from build123d import *

# Parameters (mm, degrees)
F0_W     = 19.05
F0_H     = 10.024884
F0_R     = 3.2004
F1_DEPTH = 25.4
F2_DEPTH = 19.05
F3_DEPTH = 25.4


with BuildPart() as f1:
    # F0 (on Front) → F1 (new body)
    with BuildSketch(Plane.XZ):
        with Locations((47.891052, 14.037558)):
            Rectangle(F0_W, F0_H)
        Polygon((19.316052, 0), (171.716052, 0), (171.716052, 19.05), (57.416052, 19.05), (57.416052, 9.025116), (38.366052, 9.025116), (38.366052, 19.05), (19.316052, 19.05), align=None)
        with Locations((159.016052, 10.429697)):
            Circle(F0_R, mode=Mode.SUBTRACT)
    extrude(amount=F1_DEPTH)

    # F0 (on Front) → F2 (join)
    with BuildSketch(Plane.XZ):
        with Locations((47.891052, 14.037558)):
            Rectangle(F0_W, F0_H)
    extrude(amount=F2_DEPTH)

    # F0 (on Front) → F3 (cut)
    with BuildSketch(Plane.XZ):
        with Locations((47.891052, 14.037558)):
            Rectangle(F0_W, F0_H)
    extrude(amount=F3_DEPTH, mode=Mode.SUBTRACT)


solid = f1.part
Source: CAD feature listing. Evaluate the final solid. Frame: model axes, mm. A direction names the side the tool comes from. Round coordinates to 2 decimals unless told otherwise and drop trailing zeros. Write each loop counter-clockwise with the first axis right and the second up, starting at its lowest first coordinate (ties: lowest second). Pieces come first, ordered by that corner, then holes. Notation, with made-up numbers: (76.25, 86) - (99.25, 86) arc R20 cw to (99.25, 121) - close; hole circle Ø6 at (-14.75, 89.25). An arc over 180 degrees is marked (long way). Use CSV: the item, a comma, the result in double quotes. Start each with the question number.
(1) Mould query, pull axis X, two halves, no side actions, for faces 3 (the face through (19.316, -13, 10)), 4 (the face through (155.82, -12.52, 10.57)), 5 (the face through (115, -13, 19.05)). Classes: pulls with the +X half, pulls with the -X half, needs draft (parallel to the pull), parting line crosses it, or undercut.
(2) Cut plane B-B, the plane y = -7.5. Return loops of the section in (x, z).
(3) Cut plane A-A, the plane z = 16.5. Return loops of the section in (x, y), and give its area (3 significant figures).
(4) Material intervals for probe 1 along X at (y, z) = (-2.5, 17.5); probe 2 along X at (y, z) = (-6, 11); probe 3 along X at (y, z) = (-3.5, 12.75), sorted ascending. Write a range as [from, to].
(5) First-contact query: pin 1 Ø1.5 at (x, z) = (137, 5) entering from +Y. Flat tip, straight axial feed; report the tip coordinate or a pass-through.
(6) Set-up query: faces 1 (the face through (94, 0, 10)), 2 (the face through (38.366, -13, 14)). Return all of +Z, -Z, +X, -X, +Y, -Y with unobstructed straight access to the full face (end or side cutting, diameter ignored); none if empty.
Geometry says:
1,face 3,"pulls with the -X half"
1,face 4,"undercut"
1,face 5,"needs draft"
2,outline,"(19.32, 0) - (171.72, 0) - (171.72, 19.05) - (57.42, 19.05) - (57.42, 9.03) - (38.37, 9.03) - (38.37, 19.05) - (19.32, 19.05) - close; hole circle Ø6.4 at (159.02, 10.43)"
3,outline,"(19.32, -25.4) - (38.37, -25.4) - (38.37, 0) - (19.32, 0) - close; (57.42, -25.4) - (171.72, -25.4) - (171.72, 0) - (57.42, 0) - close"
3,area,"3,390 mm²"
4,probe 1,"[19.32, 38.37], [57.42, 171.72]"
4,probe 2,"[19.32, 38.37], [57.42, 155.87], [162.17, 171.72]"
4,probe 3,"[19.32, 38.37], [57.42, 156.81], [161.22, 171.72]"
5,pin 1,"y = 0"
6,face 1,"+Z, -Z, +X, -X, +Y"
6,face 2,"+Z, +Y, -Y"
